The figure shows three views and two pictorial views of one solid part (mm, origin at its lowest corner). Answer the questions. A direction names the side the tool comes from. Coordinates: 2 decimals unless noted, no trailing zeros. Order: outer loops, then holes, each group sorted by start corner. A loop starts at its lowest first (then second) coordinate and runs counter-clockwise, first axis right, second up. Notation, with made-up numbers: (13, 76) -> (47, 76) arc R11 cw to (47, 91) -> close; hole circle Ø4 at (21.25, 16.5). An arc over 180 degrees is marked (long way). Use one line per item in the form item = value.
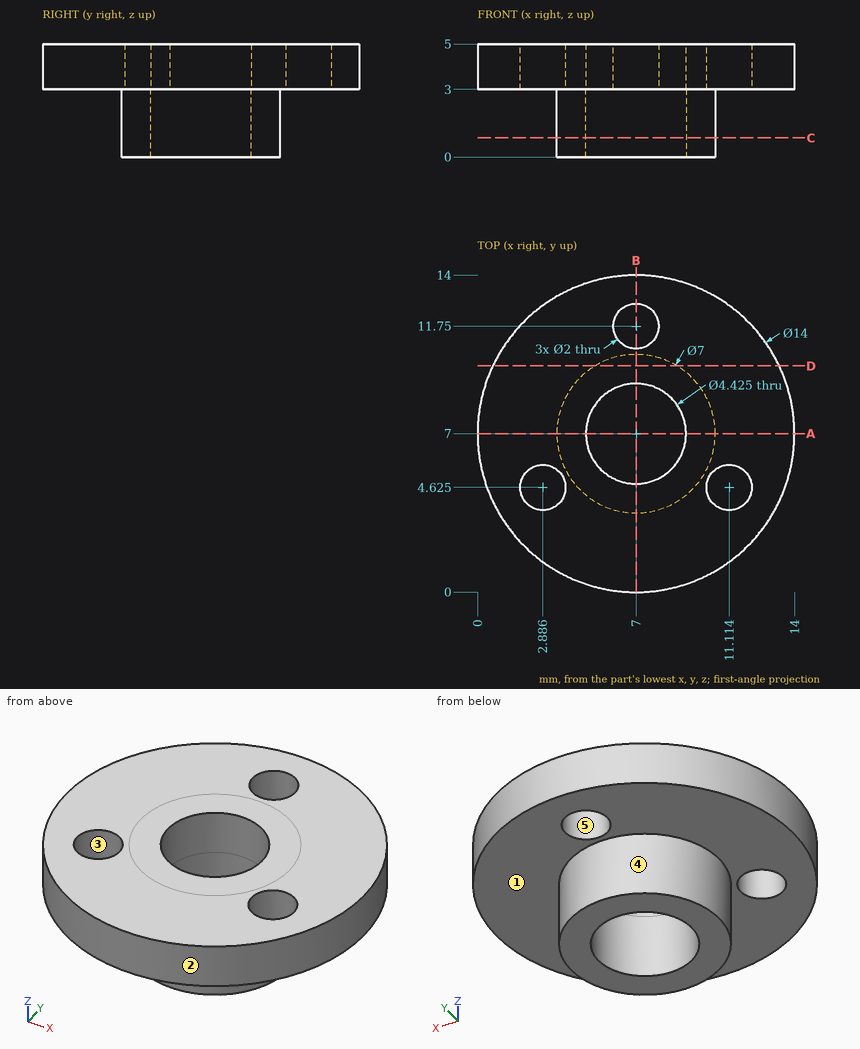
(1) Which of the six approach directions +Z, -Z, +X, -X, +Y, -Y give full straight-line access (tool end or side, diameter ignored) to the marked faces 4 and 5?
Data:
face_4 = -Z
face_5 = +Z, -Z
(2) Straight lines are drawn through the part: line 1 along X through (y, z) = (4.75, 4.1) (1 decimal); line 2 along Y through (x, z) = (7, 2.35); line 3 along Z through (x, y) = (10.75, 2.5). For each, find the intervals that lie inside material, in ascending order.
Data:
line_1 = 0.4 to 1.9, 3.9 to 10.1, 12.1 to 13.6
line_2 = 3.5 to 4.79, 9.21 to 10.5
line_3 = 3 to 5
(3) Section A-A on y = 7 is taken. Write down the section's boundary in (x, z).
Data:
outline = (0, 3) -> (3.5, 3) -> (3.5, 0) -> (4.79, 0) -> (4.79, 5) -> (0, 5) -> close; (9.21, 0) -> (10.5, 0) -> (10.5, 3) -> (14, 3) -> (14, 5) -> (9.21, 5) -> close
(4) Each of these flat-tipped pins is pushed along its axis until it touches: P1, Ø1.5, axis at x = 6.5, z = 1, coming from the -Y side; P2, Ø1.2, axis at x = 11.11, y = 4.62, coming from the +Z side; P3, Ø3, axis at y = 11.5, z = 4, coming from the -X side (1 decimal). Where does it stop, or does it pass through?
Data:
P1 = 3.5
P2 = through
P3 = 0.7
(5) The mould has two halves that part along Y. Classify the marked faces 1, 2 and 3: released by +Y, released by -Y, zero draft, split by the parting line, or undercut.
Data:
face_1 = zero draft
face_2 = split by the parting line
face_3 = undercut
(6) Section D-D on y = 10 is taken. Write down the section's boundary in (x, z) (1 decimal).
Data:
outline = (0.7, 3) -> (5.2, 3) -> (5.2, 0) -> (8.8, 0) -> (8.8, 3) -> (13.3, 3) -> (13.3, 5) -> (0.7, 5) -> close
(7) Section B-B on x = 7 is taken. Write down the section's boundary in (y, z).
Data:
outline = (0, 3) -> (3.5, 3) -> (3.5, 0) -> (4.79, 0) -> (4.79, 5) -> (0, 5) -> close; (9.21, 0) -> (10.5, 0) -> (10.5, 3) -> (10.75, 3) -> (10.75, 5) -> (9.21, 5) -> close; (12.75, 3) -> (14, 3) -> (14, 5) -> (12.75, 5) -> close
(8) Section C-C on z = 0.85 is taken. Write down the section's boundary in (x, y) (1 decimal), plus the area to 3 significant figures.
Data:
outline = circle Ø7 at (7, 7); hole circle Ø4.4 at (7, 7)
area = 23.1 mm²
